Autodesk Inventor part; units mm, degrees
ref_plane "YZ Plane" through (0, 0, 0) normal (1, 0, 0) x (0, 1, 0)
ref_plane "XZ Plane" through (0, 0, 0) normal (0, 1, 0) x (-1, 0, 0)
ref_plane "XY Plane" through (0, 0, 0) normal (0, 0, 1) x (1, 0, 0)
sketch "Sketch1" plane through (0, 0, 0) normal (0, 0, 1) x (1, 0, 0)
  line L0 (-25, 50) -> (25, 50)
  line L1 (25, 50) -> (25, -50)
  line L2 (25, -50) -> (-25, -50)
  line L3 (-25, -50) -> (-25, 50)
  line L4 (-25, 0) -> (25, 0) construction
  point P0 (0, 0)
  point P1 (0, 0)
  dimension "d0" = 50
  dimension "d1" = 100
extrude "Extrusion1" add sketch "Sketch1" along normal blind 6
sketch "Sketch2" plane through (0, 0, 6) normal (0, 0, 1) x (1, 0, 0)
  line L0 (-25, 50) -> (25, 50)
  line L1 (25, -50) -> (-25, -50)
  line L2 (0, 50) -> (0, -35) construction
  point P0 (0, 0)
  dimension "d4" = 15
hole "Hole1" at (0, -35, 6) direction (0, 0, -1) diameter 10 end through all
sketch "Sketch3" plane through (0, 0, 6) normal (0, 0, 1) x (1, 0, 0)
  line L0 (-25, 50) -> (25, 50)
  line L1 (-3.5, 30) -> (3.5, 30)
  line L2 (3.5, 30) -> (3.5, 13)
  line L3 (3.5, 13) -> (-3.5, 13)
  line L4 (-3.5, 13) -> (-3.5, 30)
  line L5 (0, 30) -> (0, 13) construction
  circle A0 centre (0, 30) radius 1.75
  circle A1 centre (0, 13) radius 1.75
  point P0 (0, 0)
  dimension "d12" = 7
  dimension "d13" = 17
  dimension "d14" = 3.5
  dimension "d15" = 3.5
  dimension "d16" = 20
extrude "Extrusion2" cut sketch "Sketch3" against normal up to next
sketch "Sketch4" plane through (0, 0, 6) normal (0, 0, 1) x (1, 0, 0)
  arc A0 (1.75, 30) -> (-1.75, 30) centre (0, 30) ccw
  line L0 (-25, 50) -> (25, 50)
  line L1 (-25, -50) -> (-25, 50)
  line L2 (10, 44) -> (25, 44)
  line L3 (25, 50) -> (25, 44)
  line L4 (10, 50) -> (25, 50)
  line L5 (10, 50) -> (10, 44)
  line L6 (-25, 44) -> (-10, 44)
  line L7 (-10, 50) -> (-10, 44)
  line L8 (-25, 50) -> (-10, 50)
  line L9 (-25, 50) -> (-25, 44)
  line L10 (0, 50) -> (0, 31.75) construction
  point P0 (0, 0)
extrude "Extrusion3" cut sketch "Sketch4" against normal up to next
properties part number "TOP"
Design review of the part built by this model. Coordinates are the model's own, in mm. A direction names the side the tool comes from. Give positions to 0.01 mm unless a question says otherwise; leave off trailing zeros. Order: outer loops, then holes, each group sorted by start corner. A loop starts at its lowest first (then second) coordinate and runs counter-clockwise, first axis right, second up.
1. Add section A-A, the plane x = 0. State the section outline as (y, z) points, then the cut area to 3 significant figures.
Solution:
outline: (-50, 0) - (-40, 0) - (-40, 6) - (-50, 6) - close; (-30, 0) - (11.25, 0) - (11.25, 6) - (-30, 6) - close; (31.75, 0) - (50, 0) - (50, 6) - (31.75, 6) - close
area: 417 mm2
2. Add section C-C, the plane z = 4.85. State the section outline as (x, y) points.
Solution:
outline: (-25, -50) - (25, -50) - (25, 44) - (10, 44) - (10, 50) - (-10, 50) - (-10, 44) - (-25, 44) - close; hole circle Ø10 at (0, -35); hole (-3.5, 13) - (-1.75, 13) arc R1.75 ccw to (1.75, 13) - (3.5, 13) - (3.5, 30) - (1.75, 30) arc R1.75 ccw to (-1.75, 30) - (-3.5, 30) - close
3. Add section D-D, the plane x = 22.5. State the section outline as (y, z) points, then the cut area to 3 significant figures.
Solution:
outline: (-50, 0) - (44, 0) - (44, 6) - (-50, 6) - close
area: 564 mm2
4. Tool access review of faces 1 (the flat face through (-3.5, 21, 3)), 2 (the flat face through (-18, 44, 3)), 3 (the flat face through (17, 44, 3)), 4 (the flat face through (0, 1, 0)): name each direction out of +Z, -Z, +X, -X, +Y, -Y from which nothing blocks a thin tool from reaching the whole face with its end or side.
Solution:
face 1: +Z, -Z
face 2: +Z, -Z, -X, +Y
face 3: +Z, -Z, +X, +Y
face 4: -Z, +X, -X, +Y, -Y
5. For pin 1 Ø8 at (x, y) = (-18, -18.5) entering from -Z; pin 2 Ø6 at (x, y) = (0, -35) entering from +Z; pin 3 Ø3 at (x, z) = (-19, 4) entering from +Y; pin 4 Ø1.8 at (y, z) = (47, 4) entering from +X, all flat-tipped, find the tip position at first contact; note any pin that passes through.
Solution:
pin 1: stops at z = 0
pin 2: passes through
pin 3: stops at y = 44
pin 4: stops at x = 10
6. Add section B-B, the plane y = -35. State the section outline as (x, z) points, then the cut area to 3 significant figures.
Solution:
outline: (-25, 0) - (-5, 0) - (-5, 6) - (-25, 6) - close; (5, 0) - (25, 0) - (25, 6) - (5, 6) - close
area: 240 mm2
7. To check wall thickness, follow L1, parallel to Y at x = 0, z = 1.3; L2, parallel to X at y = 20.5, z = 0.6; L3, parallel to Y at x = -1.5, z = 4.4. State the ranges of each line that lie inside material, in increasing order.
Solution:
L1: y = -50 to -40, -30 to 11.25, 31.75 to 50
L2: x = -25 to -3.5, 3.5 to 25
L3: y = -50 to -39.77, -30.23 to 12.1, 30.9 to 50
8. Mouldability with a two-part tool opening along Y and no side actions: class faces 5 (the flat face through (0, -50, 3)), 6 (the flat face through (3.5, 22, 3)), 7 (the flat face through (-25, -4, 3)) as +Y half, -Y half, draft (parallel to the pull), parting line (faces both ways), or undercut.
Solution:
face 5: -Y half
face 6: undercut
face 7: draft
